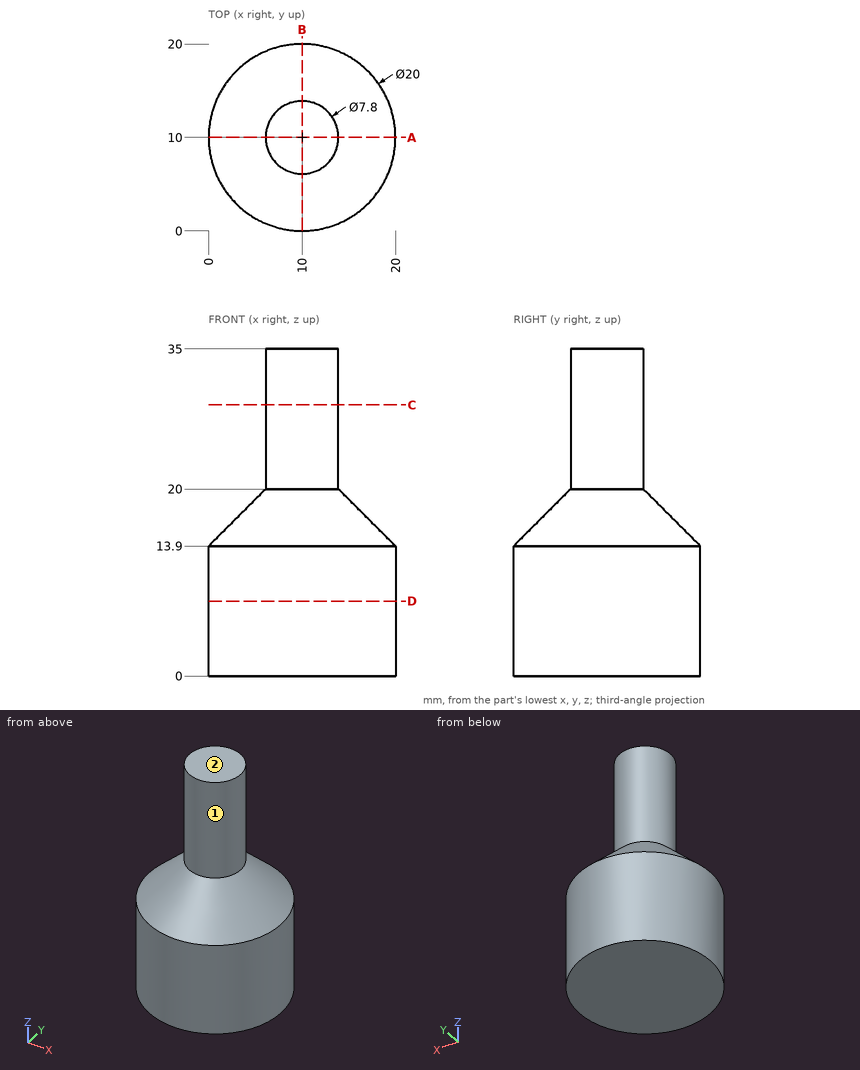
Print and shaded views of the part. All mm, measured from the part's lowest x, y and z. A direction names the side the tool comes from. Give positions to 0.01 mm unless a question says otherwise; leave off trailing zeros. Loops run counter-clockwise (first coordinate to the right, second up) from the corner with the lowest first, then second, coordinate; pieces in that order, holes last.
1) Saw through at D-D (z = 8). Write the cut outline in (x, y), plus the area to 3 significant figures.
2) Tool access for the marked faces 1 and 2: list every direction of +Z, -Z, +X, -X, +Y, -Y with a clear straight run to the whole face (end or side of a thin tool).
3) Wall check: line 1 (X direction, y = 9.75, z = 2.5); line 2 (Z direction, x = 5.5, y = 4); line 3 (X direction, y = 9.5, z = 17). Give the ranges that are in metal, low to high.
4) Flat gauge pins, fed straight in: pin 1 Ø3 at (x, y) = (4.5, 14) entering from -Z; pin 2 Ø1.5 at (x, z) = (4.5, 4) entering from -Y; pin 3 Ø6 at (x, z) = (4.5, 18) entering from +Y; pin 4 Ø10 at (y, z) = (18, 24) entering from +X. Where does each tip first touch, or does it go through?
5) Saw through at A-A (y = 10). Write the cut outline in (x, z), plus the area to 3 significant figures.
6) Saw through at C-C (z = 29). Write the cut outline in (x, y).
Answer block:
1. outline: circle Ø20 at (10, 10)
1. area: 314 mm2
2. face 1: +Z
2. face 2: +Z, +X, -X, +Y, -Y
3. line 1: x = 0 to 20
3. line 2: z = 0 to 16.4
3. line 3: x = 3.12 to 16.88
4. pin 1: stops at z = 0
4. pin 2: stops at y = 1.2
4. pin 3: stops at y = 17.51
4. pin 4: stops at x = 12.49
5. outline: (0, 0) - (20, 0) - (20, 13.9) - (13.9, 20) - (13.9, 35) - (6.1, 35) - (6.1, 20) - (0, 13.9) - close
5. area: 480 mm2
6. outline: circle Ø7.8 at (10, 10)
